Verification items for the finished model (mm, model axes). Face numbers are marked on the shaded views. Give positions to 0.01 mm unless a question says otherwise; leave off trailing zeros. Loops run counter-clockwise (first coordinate to the right, second up) from the corner with the lowest first, then second, coordinate; pieces in that order, holes last. Notation, with made-up numbers: (4, 70.5) - (62, 70.5) arc R21 cw to (62, 100.5) - close; hole circle Ø4 at (88.25, -12.75). An arc over 180 degrees is marked (long way). One line per item, written item: value. Start each with the question number.
1. Sectioned sample at C-C (x = -3). Record the cut outline in (y, z).
2. Sectioned sample at D-D (y = 4.25). Record the cut outline in (x, z).
3. Gauge pin test, flat ends, axial feed: pin 1 (1 mm diameter, centred on x = -4.5, z = -2.5, fed in from +Y); pin 2 (2.5 mm diameter, centred on x = 0, y = 0, fed in from +Z). Record the tip position at first contact, or that the pin passes through.
4. Scan lines: L1, parallel to Y at x = 0, z = -2.25 (3 decimals); L2, parallel to X at y = 0, z = -5.5 (3 decimals); L3, parallel to Y at x = -0.75, z = -3. Record each from-to range of solid material in increasing order. Write a range as [from, to].
5. Sectioned sample at A-A (y = 0). Record the cut outline in (x, z) (3 decimals), plus the area to 3 significant figures.
6. Mould release check, pull along X, two halves, no side actions. Record for the marked faces 1, 2, 3 and 4: pulls with the +X half, pulls with the -X half, needs draft (parallel to the pull), parting line crosses it, or undercut.
7. Sectioned sample at B-B (z = -5). Record the cut outline in (x, y) (3 decimals).
Solid Edge part; units mm, degrees
sketch "Sketch1" plane through (0, 0, 0) normal (0, 0, 1) x (1, 0, 0)
  line L0 (-10, 6) -> (-10, -6)
  line L1 (-10, -6) -> (-8, -6)
  line L2 (-8, -6) -> (0, -4)
  arc A0 (0, 4) -> (0, -4) centre (0, 0) cw
  line L3 (-8, 6) -> (0, 4)
  line L4 (-10, 6) -> (-8, 6)
  dimension "D1" = 10
  dimension "D2" = 10
  dimension "D3" = 8
extrude "Protrusion1" add sketch "Sketch1" against normal blind 8
hole "screw_hole" at (0, 0, 0) direction (0, 0, -1) diameter 2.75 depth 30 tip angle 118 start chamfer 0.6 start chamfer angle 45 end chamfer 0.6 end chamfer angle 45
chamfer "side_chamfers" distance 1 angle 45 6 edges at (-4, -5, 0) (4, 0, 0) (-4, 5, 0) (-4, -5, -8) (4, 0, -8) (-4, 5, -8)
properties material "Polyethylene, low density"
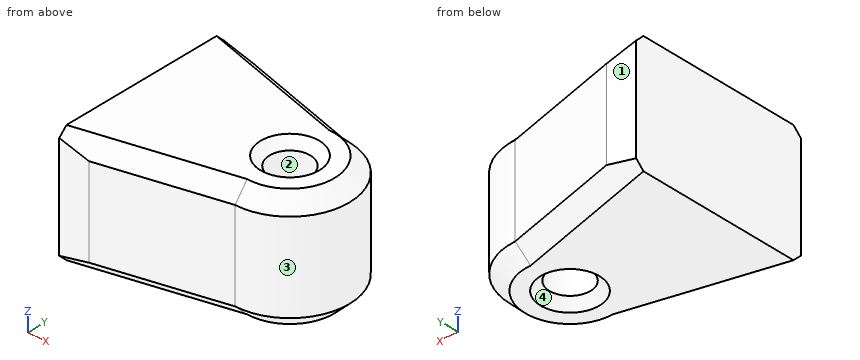
Results are:
1. outline: (-4.75, -7) - (-3.72, -8) - (3.72, -8) - (4.75, -7) - (4.75, -1) - (3.72, 0) - (-3.72, 0) - (-4.75, -1) - close
2. outline: (-10, -8) - (-5.12, -8) - (-1, -7) - (-1, -1) - (-5.12, 0) - (-10, 0) - close
3. pin 1: stops at y = 5.25
3. pin 2: passes through
4. L1: y = [-4, -1.375], [1.375, 4]
4. L2: x = [-10, -1.375], [1.375, 4]
4. L3: y = [-4.19, -1.15], [1.15, 4.19]
5. outline: (-10, -8) - (-1.975, -8) - (-1.375, -7.4) - (-1.375, -0.6) - (-1.975, 0) - (-10, 0) - close; (1.375, -7.4) - (1.975, -8) - (3, -8) - (4, -7) - (4, -1) - (3, 0) - (1.975, 0) - (1.375, -0.6) - close
5. area: 88.3 mm^2
6. face 1: needs draft
6. face 2: undercut
6. face 3: pulls with the +X half
6. face 4: undercut
7. outline: (-10, -6) - (-8, -6) - (0, -4) arc R4 ccw to (0, 4) - (-8, 6) - (-10, 6) - close; hole circle Ø2.75 at (0, 0)
